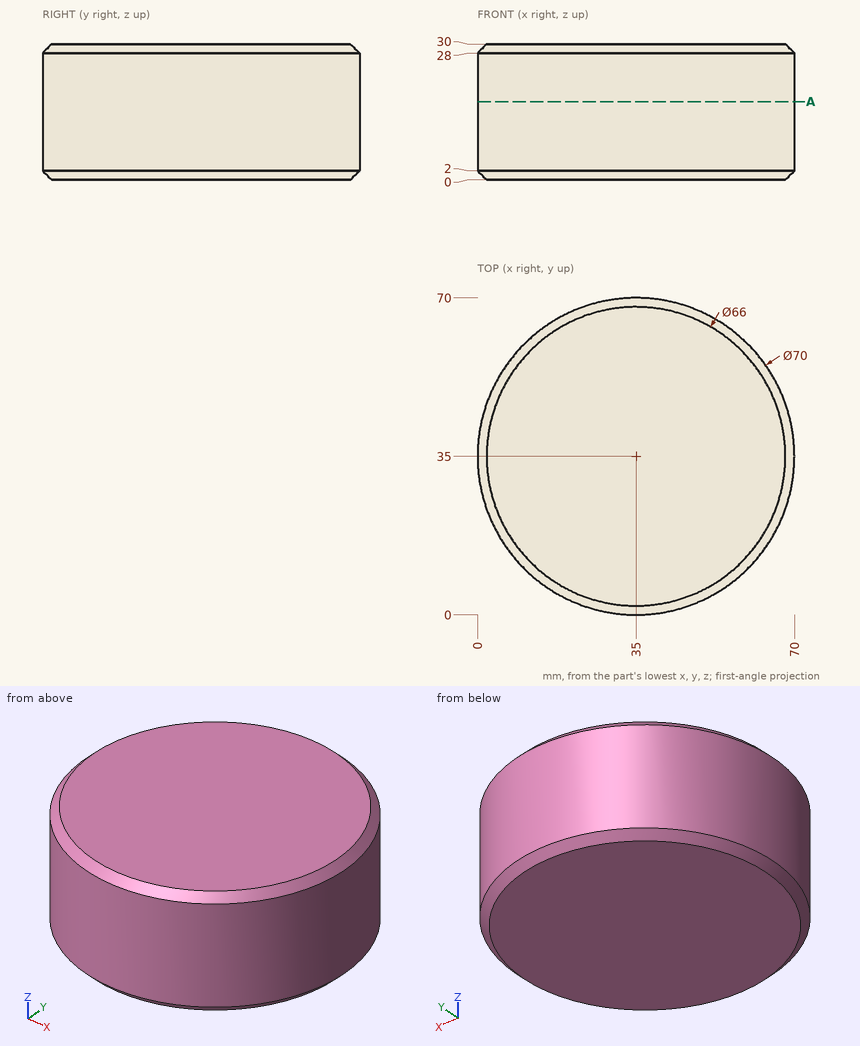
Design review of the part shown in the three views and the two pictorial views. Dimensions are in mm from the part's minimum x, y and z. Give positions to 0.01 mm unless a question says otherwise; leave off trailing zeros. Loops run counter-clockwise (first coordinate to the right, second up) from the corner with the lowest first, then second, coordinate; pieces in that order, holes last. Notation, with made-up numbers: (14, 54.5) -> (67, 54.5) arc R13 cw to (67, 62.5) -> close; hole circle Ø1 at (-3.75, 49.5). An arc over 180 degrees is marked (long way). One line per question, with ' | ' between items.
1) Insertion check: pin 1 Ø8 at (x, z) = (53, 17) entering from +Y; pin 2 Ø3 at (x, y) = (13, 27.5) entering from -Z; pin 3 Ø1 at (x, z) = (60.5, 14.5) entering from -Y; pin 4 Ø10 at (y, z) = (47.5, 16.5) entering from +X. Each pin has a flat end and moves straight along its axis. Give the tip position at first contact, or say it passes through.
Resolved:
pin 1: stops at y = 67.08 | pin 2: stops at z = 0 | pin 3: stops at y = 10.51 | pin 4: stops at x = 69.19
2) To check wall thickness, follow probe 1 along Y at (x, z) = (62, 9); probe 2 along X at (y, z) = (43, 11.25); probe 3 along Y at (x, z) = (4.5, 13.5). State the ranges of each line that lie inside material, in increasing order.
Resolved:
probe 1: y = 12.73 to 57.27 | probe 2: x = 0.93 to 69.07 | probe 3: y = 17.83 to 52.17
3) We need section A-A (z = 17.25). Write out the cut boundary in (x, y), plus the area to 3 significant figures.
Resolved:
outline: circle Ø70 at (35, 35) | area: 3,850 mm2
